from build123d import *

# Parameters (mm, degrees)
SCHIZZO1_R                   = 115
ESTRUSIONE_ESTRUSIONE1_DEPTH = 75
TAGLIO_ESTRUSIONE1_REACH     = 77
SCHIZZO3_W                   = 60
SCHIZZO3_H                   = 60
TAGLIO_ESTRUSIONE2_DEPTH     = 15
SCHIZZO4_W                   = 50
SCHIZZO4_H                   = 70
TAGLIO_ESTRUSIONE3_DEPTH     = 25
SCHIZZO5_R                   = 5
TAGLIO_ESTRUSIONE4_DEPTH     = 76
SCHIZZO6_W                   = 45
SCHIZZO6_H                   = 45
TAGLIO_ESTRUSIONE5_DEPTH     = 12


with BuildPart() as part:
    # Schizzo1 → Estrusione-Estrusione1 (new body)
    with BuildSketch(Plane.XY):
        Circle(SCHIZZO1_R)
    extrude(amount=ESTRUSIONE_ESTRUSIONE1_DEPTH)

    # Schizzo2 → Taglio-Estrusione1 (cut, up to next)
    with BuildSketch(Plane(origin=(0, 0, 0), x_dir=(-1, 0, 0), z_dir=(0, 0, -1)), mode=Mode.PRIVATE) as taglio_estrusione1_sk1:
        with BuildLine():
            Line((58.610597259, -81.721507315), (66.78904506, -93.617431389))
            ThreePointArc((66.78904506, -93.617431389), (65.150814632, -94.764821283), (63.492877363, -95.883546681))
            Line((63.492877363, -95.883546681), (55.314429562, -83.987622606))
            ThreePointArc((55.314429562, -83.987622606), (52.733884708, -76.703832303), (58.610597259, -81.721507315))
        make_face()
    taglio_estrusione1_tool1 = extrude(taglio_estrusione1_sk1.sketch, amount=-TAGLIO_ESTRUSIONE1_REACH, mode=Mode.PRIVATE) & part.part
    add(taglio_estrusione1_tool1.solids().sort_by_distance((-58.254036, -84.733143, 0))[0], mode=Mode.SUBTRACT)
    # Schizzo2 → Taglio-Estrusione1 (cut, up to next)
    with BuildSketch(Plane(origin=(0, 0, 0), x_dir=(-1, 0, 0), z_dir=(0, 0, -1)), mode=Mode.PRIVATE) as taglio_estrusione1_sk2:
        with BuildLine():
            Line((81.721507315, 58.610597259), (93.617431389, 66.78904506))
            ThreePointArc((93.617431389, 66.78904506), (94.764821283, 65.150814632), (95.883546681, 63.492877363))
            Line((95.883546681, 63.492877363), (83.987622606, 55.314429562))
            ThreePointArc((83.987622606, 55.314429562), (76.703832303, 52.733884708), (81.721507315, 58.610597259))
        make_face()
    taglio_estrusione1_tool2 = extrude(taglio_estrusione1_sk2.sketch, amount=-TAGLIO_ESTRUSIONE1_REACH, mode=Mode.PRIVATE) & part.part
    add(taglio_estrusione1_tool2.solids().sort_by_distance((-84.733143, 58.254036, 0))[0], mode=Mode.SUBTRACT)
    # Schizzo2 → Taglio-Estrusione1 (cut, up to next)
    with BuildSketch(Plane(origin=(0, 0, 0), x_dir=(-1, 0, 0), z_dir=(0, 0, -1)), mode=Mode.PRIVATE) as taglio_estrusione1_sk3:
        with BuildLine():
            Line((-58.610597259, 81.721507315), (-66.78904506, 93.617431389))
            ThreePointArc((-66.78904506, 93.617431389), (-65.150814632, 94.764821283), (-63.492877363, 95.883546681))
            Line((-63.492877363, 95.883546681), (-55.314429562, 83.987622606))
            ThreePointArc((-55.314429562, 83.987622606), (-52.733884708, 76.703832303), (-58.610597259, 81.721507315))
        make_face()
    taglio_estrusione1_tool3 = extrude(taglio_estrusione1_sk3.sketch, amount=-TAGLIO_ESTRUSIONE1_REACH, mode=Mode.PRIVATE) & part.part
    add(taglio_estrusione1_tool3.solids().sort_by_distance((58.254036, 84.733143, 0))[0], mode=Mode.SUBTRACT)
    # Schizzo2 → Taglio-Estrusione1 (cut, up to next)
    with BuildSketch(Plane(origin=(0, 0, 0), x_dir=(-1, 0, 0), z_dir=(0, 0, -1)), mode=Mode.PRIVATE) as taglio_estrusione1_sk4:
        with BuildLine():
            Line((-81.721507315, -58.610597259), (-93.617431389, -66.78904506))
            ThreePointArc((-93.617431389, -66.78904506), (-94.764821283, -65.150814632), (-95.883546681, -63.492877363))
            Line((-95.883546681, -63.492877363), (-83.987622606, -55.314429562))
            ThreePointArc((-83.987622606, -55.314429562), (-76.703832303, -52.733884708), (-81.721507315, -58.610597259))
        make_face()
    taglio_estrusione1_tool4 = extrude(taglio_estrusione1_sk4.sketch, amount=-TAGLIO_ESTRUSIONE1_REACH, mode=Mode.PRIVATE) & part.part
    add(taglio_estrusione1_tool4.solids().sort_by_distance((84.733143, -58.254036, 0))[0], mode=Mode.SUBTRACT)

    # Schizzo3 → Taglio-Estrusione2 (cut)
    with BuildSketch(Plane(origin=(0, 0, 0), x_dir=(-1, 0, 0), z_dir=(0, 0, -1))):
        with Locations((-35, 0)):
            Rectangle(SCHIZZO3_W, SCHIZZO3_H)
    extrude(amount=-TAGLIO_ESTRUSIONE2_DEPTH, mode=Mode.SUBTRACT)

    # Schizzo4 → Taglio-Estrusione3 (cut)
    with BuildSketch(Plane(origin=(0, 0, 0), x_dir=(-1, 0, 0), z_dir=(0, 0, -1))):
        with Locations((40, 0)):
            Rectangle(SCHIZZO4_W, SCHIZZO4_H)
    extrude(amount=-TAGLIO_ESTRUSIONE3_DEPTH, mode=Mode.SUBTRACT)

    # Schizzo5 → Taglio-Estrusione4 (cut, through all)
    with BuildSketch(Plane(origin=(0, 0, 0), x_dir=(-1, 0, 0), z_dir=(0, 0, -1))):
        with Locations((0, 55)):
            Circle(SCHIZZO5_R)
    extrude(amount=-TAGLIO_ESTRUSIONE4_DEPTH, mode=Mode.SUBTRACT)

    # Schizzo6 → Taglio-Estrusione5 (cut)
    with BuildSketch(Plane(origin=(0, 0, 0), x_dir=(-1, 0, 0), z_dir=(0, 0, -1))):
        with Locations((0, 84.5)):
            Rectangle(SCHIZZO6_W, SCHIZZO6_H)
    extrude(amount=-TAGLIO_ESTRUSIONE5_DEPTH, mode=Mode.SUBTRACT)


solid = part.part
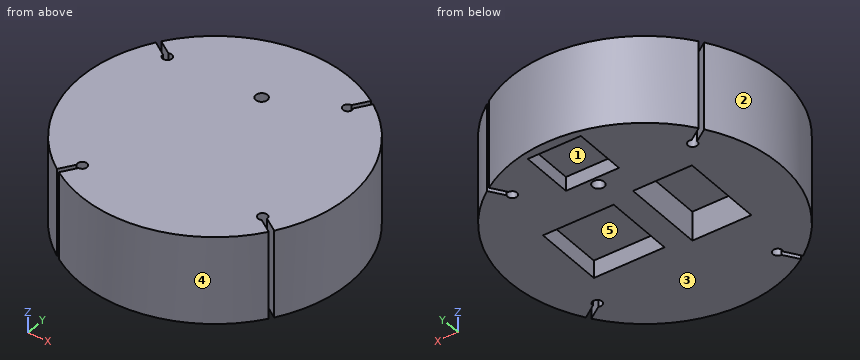
Geometry check sheet. Reference: the model listing, model coordinates, mm. Face numbers are marked on the shaded views. A direction names the side the tool comes from. Give positions to 0.01 mm unless a question says otherwise; leave off trailing zeros. Order: outer loops, then holes, each group sorted by start corner. A loop starts at its lowest first (then second) coordinate and runs counter-clockwise, first axis right, second up.
1. Scan lines: line 1 (Y direction, x = 0, z = 38); line 2 (X direction, y = 0, z = 30); line 3 (Z direction, x = -15.5, y = 105). Record each from-to range of solid material in increasing order.
Completed:
line 1: y = -115 to 50, 60 to 115
line 2: x = -115 to 115
line 3: z = 12 to 75
2. Sectioned sample at D-D (y = -24). Record the boundary of the cut face in (x, z), then the cut area to 3 significant figures.
Completed:
outline: (-112.47, 0) - (-65, 0) - (-65, 25) - (-15, 25) - (-15, 0) - (5, 0) - (5, 15) - (65, 15) - (65, 0) - (112.47, 0) - (112.47, 75) - (-112.47, 75) - close
area: 14,700 mm2
3. Sectioned sample at A-A (x = 0). Record the boundary of the cut face in (y, z).
Completed:
outline: (-115, 0) - (50, 0) - (50, 75) - (-115, 75) - close; (60, 0) - (62, 0) - (62, 12) - (107, 12) - (107, 0) - (115, 0) - (115, 75) - (60, 75) - close
4. Sectioned sample at B-B (z = 33). Record the boundary of the cut face in (x, y).
Completed:
outline: (-95.88, 63.49) arc R115 ccw to (-66.79, -93.62) - (-58.61, -81.72) arc R4 cw (long way) to (-55.31, -83.99) - (-63.49, -95.88) arc R115 ccw to (93.62, -66.79) - (81.72, -58.61) arc R4 cw (long way) to (83.99, -55.31) - (95.88, -63.49) arc R115 ccw to (66.79, 93.62) - (58.61, 81.72) arc R4 cw (long way) to (55.31, 83.99) - (63.49, 95.88) arc R115 ccw to (-93.62, 66.79) - (-81.72, 58.61) arc R4 cw (long way) to (-83.99, 55.31) - close; hole circle Ø10 at (0, 55)
5. Draft check along Y on the marked faces 3, 4 and 5. Enter one of: pulls with the +Y half, pulls with the -Y half, needs draft (parallel to the pull), parting line crosses it, or undercut.
Completed:
face 3: needs draft
face 4: pulls with the -Y half
face 5: undercut
6. Access from +Z, -Z, +X, -X, +Y, -Y to the whole of each face (thin tool, end or side, straight path). Record for the marked faces 1 and 2.
Completed:
face 1: -Z
face 2: +Z, -Z, -X
7. Sectioned sample at C-C (z = 5.5). State how many separate pieces and enclosed holes the cut face has, then the cut area to 3 significant figures.
Completed:
separate pieces: 1
enclosed holes: 4
area: 31,900 mm2
8. Depth check by flat-ended pin: pin 1 (4 mm diameter, centred on x = 86.5, z = 25, fed in from -Y); pin 2 (3 mm diameter, centred on x = -72.5, z = 22, fed in from +Y); pin 3 (8 mm diameter, centred on x = 2.5, z = 47.5, fed in from +Y). Enter the tip coordinate at first touch or a pass-through.
Completed:
pin 1: stops at y = -78
pin 2: stops at y = 90.47
pin 3: stops at y = 115
